Work out the finished part from the listing and answer in its coordinate system (mm). Coordinates: 2 decimals unless noted, no trailing zeros. Loops run counter-clockwise (first coordinate to the right, second up) from the corner with the lowest first, then second, coordinate; pieces in that order, holes last.
```python
from build123d import *

# Parameters (mm, degrees)
SKETCH_1_R      = 2.5
EXTRUDE_1_DEPTH = 2
FILLET_1_R      = 6


with BuildPart() as part:
    # 草圖1 → 擠出1 (new body)
    with BuildSketch(Plane.XY):
        Polygon((21, 0), (21, 21), (0, 21), (0, 221), (34.5, 221), (47.301071766, 227.522471846), (227.522471846, 47.301071766), (222.528576348, 37.5), (221, 34.5), (221, 21), (221, 0), align=None)
        with Locations((11.5, 46)):
            Circle(SKETCH_1_R, mode=Mode.SUBTRACT)
        with Locations((11.5, 131)):
            Circle(SKETCH_1_R, mode=Mode.SUBTRACT)
        with Locations((11.5, 206)):
            Circle(SKETCH_1_R, mode=Mode.SUBTRACT)
        with Locations((46, 11.5)):
            Circle(SKETCH_1_R, mode=Mode.SUBTRACT)
        with Locations((131, 11.5)):
            Circle(SKETCH_1_R, mode=Mode.SUBTRACT)
        with Locations((206, 11.5)):
            Circle(SKETCH_1_R, mode=Mode.SUBTRACT)
    extrude(amount=EXTRUDE_1_DEPTH)

    # 圓角1
    fillet_1_edges = [part.edges().sort_by_distance(p)[0] for p in [
        (0, 221, 1),
        (34.5, 221, 1),
        (47.301071766, 227.522471846, 1),
        (227.522471846, 47.301071766, 1),
        (221, 34.5, 1),
        (221, 0, 1),
    ]]
    fillet(fillet_1_edges, radius=FILLET_1_R)


solid = part.part
```
1. A cutting plane is placed at B-B, the plane x = 17.5. Give the vertices of the cut face in (y, z).
2. Straight lines are drawn through the part: probe 1 along Y at (x, z) = (11.5, 1.5); probe 2 along X at (y, z) = (131, 1.25); probe 3 along X at (y, z) = (32.5, 1.7). For each, find the intervals that lie inside material, in ascending order.
3. A cutting plane is placed at C-C, the plane y = 193. Give the vertices of the cut face in (x, z).
4. Each of these flat-tipped pins is pushed along its axis until it touches: P1, Ø1, axis at y = 21, z = 1, coming from the +X side; P2, Ø4, axis at x = 11.5, y = 131, coming from the -Z side; P3, Ø1, axis at x = 21, z = 0.5, coming from the +Y side; P4, Ø0.6, axis at y = 7, z = 1, coming from the -X side. Where does it stop, or does it pass through?
5. A cutting plane is placed at A-A, the plane z = 0.3. Give the vertices of the cut face in (x, y), then the cut area to 3 significant figures.
6. Determine the mould class of faces 1 (the cylindrical face through (133.31, 10.54, 0.99)), 2 (the cylindrical face through (48.31, 10.54, 0.99)), 3 (the flat face through (90, 90, 0)), 4 (the cylindrical face through (1.711, 219.196, 1.014)) for opening direction Y: released by +Y, released by -Y, zero draft, split by the parting line, or undercut.
Answers below:
1. outline: (21, 0) - (221, 0) - (221, 2) - (21, 2) - close
2. probe 1: y = 21 to 43.5, 48.5 to 128.5, 133.5 to 203.5, 208.5 to 221
2. probe 2: x = 0 to 9, 14 to 143.82
2. probe 3: x = 0 to 221
3. outline: (0, 0) - (81.82, 0) - (81.82, 2) - (0, 2) - close
4. P1: stops at x = 221
4. P2: passes through
4. P3: stops at y = 221
4. P4: stops at x = 21
5. outline: (0, 21) - (21, 21) - (21, 0) - (215, 0) arc R6 ccw to (221, 6) - (221, 33.06) arc R6 cw to (221.65, 35.78) - (225.54, 43.42) arc R6 ccw to (224.44, 50.38) - (50.38, 224.44) arc R6 ccw to (43.42, 225.54) - (35.78, 221.65) arc R6 cw to (33.06, 221) - (6, 221) arc R6 ccw to (0, 215) - close; hole circle Ø5 at (11.5, 46); hole circle Ø5 at (11.5, 131); hole circle Ø5 at (11.5, 206); hole circle Ø5 at (46, 11.5); hole circle Ø5 at (131, 11.5); hole circle Ø5 at (206, 11.5)
5. area: 34,400 mm2
6. face 1: undercut
6. face 2: undercut
6. face 3: zero draft
6. face 4: released by +Y
